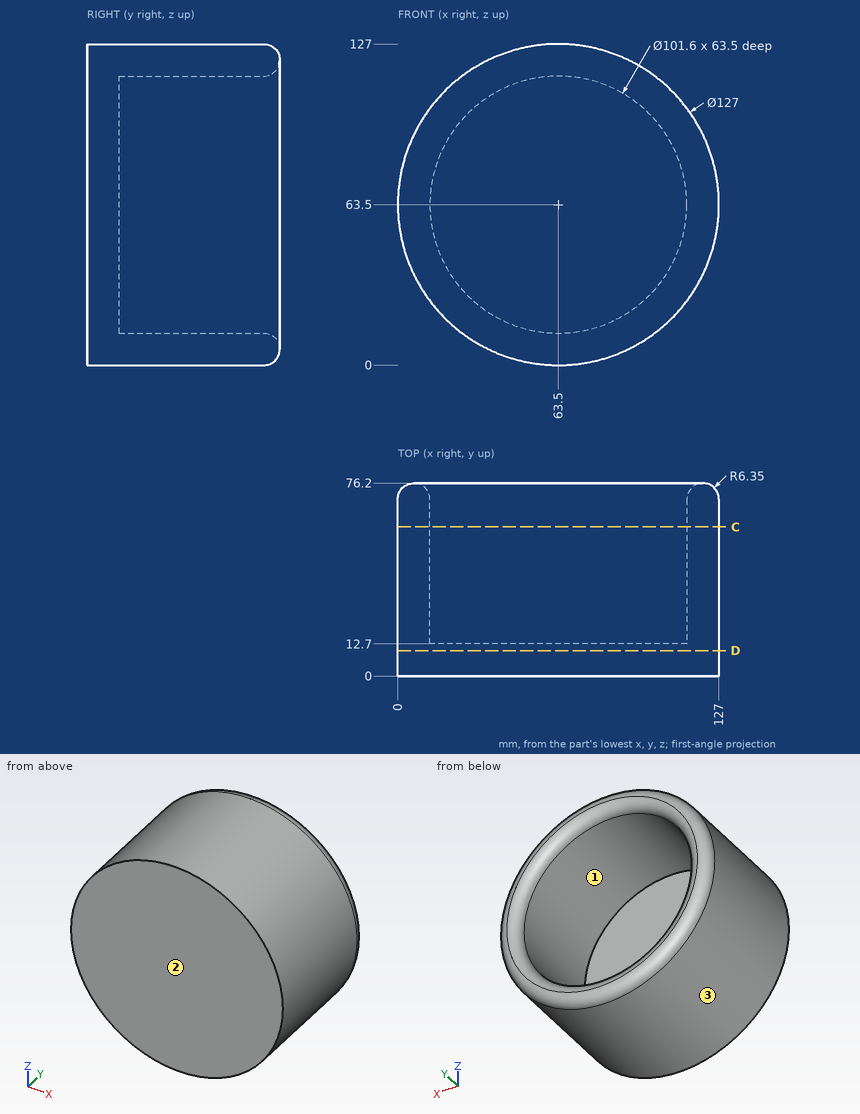
Source: three-view drawing plus pictorial views. Frame: mm from the lowest corner of the part. Give positions to 0.01 mm unless a question says otherwise; leave off trailing zeros. Write each loop counter-clockwise with the first axis right and the second up, starting at its lowest first coordinate (ties: lowest second). Pieces come first, ordered by that corner, then holes.
(1) Cut plane C-C, the plane y = 59. Return loops of the section in (x, z).
(2) Mould query, pull axis X, two halves, no side actions, for the marked faces 1, 2 and 3. Classes: released by +X, released by -X, zero draft, split by the parting line, or undercut.
(3) Ray query, line 1 (X direction, y = 33, z = 63); line 2 (Y direction, x = 59, z = 95). Return the intervals inside material, ascending.
(4) First-contact query: P1, Ø3, axis at x = 114, y = 42, coming from the -Z side; P2, Ø3, axis at x = 41.5, z = 18.5, coming from the +Y side; P3, Ø10, axis at y = 39, z = 86.5, coming from the +X side; P4, Ø5, axis at x = 103.5, z = 27.5, coming from the -Y side. Flat tips, straight axial feed; report the tip coordinate or a pass-through.
(5) Cut plane D-D, the plane y = 10. Return loops of the section in (x, z).
Values follow:
1. outline: circle Ø127 at (63.5, 63.5); hole circle Ø101.6 at (63.5, 63.5)
2. face 1: undercut
2. face 2: zero draft
2. face 3: split by the parting line
3. line 1: x = 0 to 12.7, 114.3 to 127
3. line 2: y = 0 to 12.7
4. P1: stops at z = 23.11
4. P2: stops at y = 72.92
4. P3: stops at x = 124.4
4. P4: stops at y = 0
5. outline: circle Ø127 at (63.5, 63.5)
